Read the model definition and answer for the solid it produces. Units are mm, in the model's axes. Give positions to 0.01 mm unless a question says otherwise; leave off trailing zeros.
Autodesk Inventor part; units mm, degrees
ref_plane "YZ Plane" through (0, 0, 0) normal (1, 0, 0) x (0, 1, 0)
ref_plane "XZ Plane" through (0, 0, 0) normal (0, 1, 0) x (-1, 0, 0)
ref_plane "XY Plane" through (0, 0, 0) normal (0, 0, 1) x (1, 0, 0)
sketch "Sketch1" plane through (0, 0, 0) normal (0, 0, 1) x (1, 0, 0)
  line L0 (86.5491, 25.4876) -> (86.5491, 28.0676)
  line L1 (86.5491, 28.0676) -> (86.5491, 25.4876)
  line L2 (73.8491, 25.4876) -> (86.5491, 25.4876)
  line L3 (86.5491, 25.4876) -> (73.8491, 25.4876)
  line L4 (86.5491, 28.0676) -> (217.6691, 28.0676)
  line L5 (217.6691, 28.0676) -> (86.5491, 28.0676)
  line L6 (217.6691, 28.0676) -> (217.6691, -18.6554)
  line L7 (217.6691, -18.6554) -> (217.6691, 28.0676)
  line L8 (86.5491, -18.6554) -> (217.6691, -18.6554)
  line L9 (217.6691, -18.6554) -> (86.5491, -18.6554)
  line L10 (-230.8205, -18.6554) -> (-230.8205, 28.0676)
  line L11 (-230.8205, 28.0676) -> (-230.8205, -18.6554)
  line L12 (-230.8205, 28.0676) -> (-230.8205, -18.6554)
  line L13 (-230.8205, -18.6554) -> (-230.8205, 28.0676)
  line L14 (-15.0509, -16.0754) -> (-15.0509, -18.6554)
  line L15 (-15.0509, -18.6554) -> (-15.0509, -16.0754)
  line L16 (-2.3509, 25.4876) -> (-2.3509, 28.0676)
  line L17 (-2.3509, 28.0676) -> (-2.3509, 25.4876)
  line L18 (-15.0509, 25.4876) -> (-2.3509, 25.4876)
  line L19 (-2.3509, 25.4876) -> (-15.0509, 25.4876)
  line L20 (-15.0509, 28.0676) -> (-15.0509, 25.4876)
  line L21 (-15.0509, 25.4876) -> (-15.0509, 28.0676)
  line L22 (-2.3509, -16.0754) -> (-15.0509, -16.0754)
  line L23 (-15.0509, -16.0754) -> (-2.3509, -16.0754)
  line L24 (-15.0509, 25.4876) -> (-15.0509, 28.0676)
  line L25 (-15.0509, 28.0676) -> (-15.0509, 25.4876)
  line L26 (-15.0509, -18.6554) -> (-15.0509, -16.0754)
  line L27 (-15.0509, -16.0754) -> (-15.0509, -18.6554)
  line L28 (-2.3509, 25.4876) -> (-15.0509, 25.4876)
  line L29 (-15.0509, 25.4876) -> (-2.3509, 25.4876)
  line L30 (-15.0509, -16.0754) -> (-2.3509, -16.0754)
  line L31 (-2.3509, -16.0754) -> (-15.0509, -16.0754)
  line L32 (-230.8205, 28.0676) -> (-15.0509, 28.0676)
  line L33 (-15.0509, 28.0676) -> (-230.8205, 28.0676)
  line L34 (-15.0509, 28.0676) -> (-230.8205, 28.0676)
  line L35 (-230.8205, 28.0676) -> (-15.0509, 28.0676)
  line L36 (-230.8205, -18.6554) -> (-15.0509, -18.6554)
  line L37 (-230.8205, -18.6554) -> (-15.0509, -18.6554)
  line L38 (-15.0509, -18.6554) -> (-230.8205, -18.6554)
  line L39 (-15.0509, -18.6554) -> (-230.8205, -18.6554)
  line L40 (-2.3509, -18.6554) -> (-2.3509, -16.0754)
  line L41 (73.8491, 28.0676) -> (73.8491, 25.4876)
  line L42 (73.8491, 25.4876) -> (73.8491, 28.0676)
  line L43 (-2.3509, 28.0676) -> (73.8491, 28.0676)
  line L44 (73.8491, 28.0676) -> (-2.3509, 28.0676)
  line L45 (86.5491, -18.6554) -> (86.5491, -16.0754)
  line L46 (86.5491, -16.0754) -> (86.5491, -18.6554)
  line L47 (86.5491, -16.0754) -> (73.8491, -16.0754)
  line L48 (73.8491, -16.0754) -> (86.5491, -16.0754)
  line L49 (-2.3509, -16.0754) -> (-2.3509, -18.6554)
  line L50 (-2.3509, 28.0676) -> (-2.3509, 25.4876)
  line L51 (-2.3509, 25.4876) -> (-2.3509, 28.0676)
  line L52 (-2.3509, -16.0754) -> (-2.3509, -18.6554)
  line L53 (-2.3509, -18.6554) -> (-2.3509, -16.0754)
  line L54 (73.8491, -18.6554) -> (-2.3509, -18.6554)
  line L55 (-2.3509, -18.6554) -> (73.8491, -18.6554)
  line L56 (-2.3509, -18.6554) -> (73.8491, -18.6554)
  line L57 (73.8491, -18.6554) -> (-2.3509, -18.6554)
  line L58 (73.8491, 28.0676) -> (-2.3509, 28.0676)
  line L59 (-2.3509, 28.0676) -> (73.8491, 28.0676)
  line L60 (73.8491, -16.0754) -> (73.8491, -18.6554)
  line L61 (73.8491, -18.6554) -> (73.8491, -16.0754)
  line L62 (73.8491, -18.6554) -> (73.8491, -16.0754)
  line L63 (73.8491, -16.0754) -> (73.8491, -18.6554)
  line L64 (73.8491, -16.0754) -> (86.5491, -16.0754)
  line L65 (86.5491, -16.0754) -> (73.8491, -16.0754)
  line L66 (86.5491, 25.4876) -> (73.8491, 25.4876)
  line L67 (73.8491, 25.4876) -> (86.5491, 25.4876)
  line L68 (73.8491, 25.4876) -> (73.8491, 28.0676)
  line L69 (73.8491, 28.0676) -> (73.8491, 25.4876)
  line L70 (86.5491, -16.0754) -> (86.5491, -18.6554)
  line L71 (86.5491, -18.6554) -> (86.5491, -16.0754)
  line L72 (217.6691, 28.0676) -> (86.5491, 28.0676)
  line L73 (86.5491, 28.0676) -> (217.6691, 28.0676)
  line L74 (217.6691, -18.6554) -> (217.6691, 28.0676)
  line L75 (217.6691, 28.0676) -> (217.6691, -18.6554)
  line L76 (86.5491, 28.0676) -> (86.5491, 25.4876)
  line L77 (86.5491, 25.4876) -> (86.5491, 28.0676)
  line L78 (86.5491, -18.6554) -> (217.6691, -18.6554)
  line L79 (217.6691, -18.6554) -> (86.5491, -18.6554)
  point P0 (0, 0)
extrude "Extrusion1" add sketch "Sketch1" along normal blind 2.5
move faces "Move1" translate (23, 0, 0) faces at (217.6691, -3.081, 0.8333)
move faces "Move2" translate (2, 0, 0) faces at (240.6691, 12.4933, 1.6667)
sketch "Sketch2" plane through (0, 0, 2.5) normal (0, 0, 1) x (1, 0, 0)
  line L0 (-83.3964, 28.0676) -> (-230.8205, 28.0676)
  line L1 (-230.8205, 28.0676) -> (-230.8205, -18.6554)
  line L2 (-230.8205, -18.6554) -> (-83.3964, -18.6554)
  line L3 (-83.3964, -18.6554) -> (-83.3964, 28.0676)
extrude "Extrusion2" cut sketch "Sketch2" against normal blind 10
sketch "Sketch4" plane through (-83.3964, -18.6554, 2.5) normal (-1, 0, 0) x (0, 0, 1)
  line L0 (-2.5, 0) -> (-2.5, 46.723)
  line L1 (-2.5, 46.723) -> (0, 46.723)
  line L2 (0, 46.723) -> (0, 0)
  line L3 (0, 0) -> (-2.5, 0)
  point P0 (-2.5, 18.6554)
extrude "Extrusion3" add sketch "Sketch4" along normal blind 75
sketch "Sketch5" plane through (242.6691, -18.6554, 0) normal (1, 0, 0) x (0, 0, -1)
  line L0 (-2.5, 0) -> (-2.5, 46.723)
  line L1 (0, 46.723) -> (-2.5, 46.723)
  line L2 (0, 0) -> (0, 46.723)
  line L3 (0, 0) -> (-2.5, 0)
  point P0 (0, 18.6554)
extrude "Extrusion4" add sketch "Sketch5" along normal blind 100
sketch "Sketch6" plane through (-158.3964, -18.6554, 2.5) normal (-1, 0, 0) x (0, 0, 1)
  line L0 (-2.5, 46.723) -> (-2.5, 0)
  line L1 (0, 0) -> (0, 46.723)
  line L2 (0, 46.723) -> (-2.5, 46.723)
  line L3 (-2.5, 0) -> (0, 0)
  point P0 (-2.5, 18.6554)
extrude "Extrusion5" cut sketch "Sketch6" against normal blind 75
properties part number "New base"
1) Given pin 1 (0.8 mm diameter, centred on x = -9.5, z = 1.5, fed in from +Y); pin 2 (5 mm diameter, centred on x = 210, y = 9.5, fed in from -Z); pin 3 (1.2 mm diameter, centred on x = 82.5, z = 1, fed in from -Y), each flat-ended and moving along its own axis, determine where each tip first touches the part or whether it passes through.
Final values:
pin 1: stops at y = 25.49
pin 2: stops at z = 0
pin 3: stops at y = -16.08
2) For a pull along Z with two mould halves and no side action, classify faces 1 (the face through (127, 4, 0)), 2 (the face through (127, 4, 2.5)) as released by +Z, released by -Z, zero draft, split by the parting line, or undercut.
Final values:
face 1: released by -Z
face 2: released by +Z
3) Consider L1, parallel to Y at x = -12.5, z = 0.5. Determine where the line is inside the solid, lowest interval first.
Final values:
L1: y = -16.08 to 25.49
